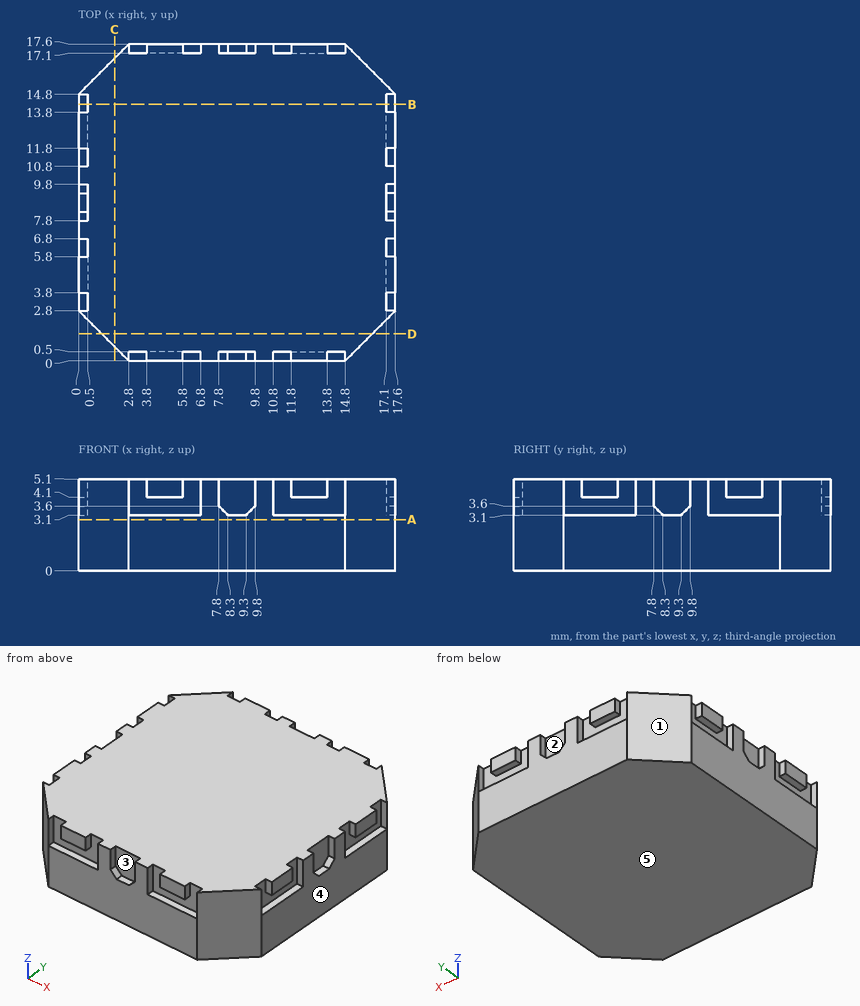
Geometry check sheet. Reference: drawing and pictorial views, mm from the part's lowest x, y, z. A direction names the side the tool comes from. Give positions to 0.01 mm unless a question says otherwise; leave off trailing zeros. Loops run counter-clockwise (first coordinate to the right, second up) from the corner with the lowest first, then second, coordinate; pieces in that order, holes last. Notation, with made-up numbers: (51.25, -10) - (59.25, -10) arc R11 cw to (59.25, 5) - close; hole circle Ø5 at (-20.5, 23). An arc over 180 degrees is marked (long way). One line per question, with ' | ' between items. Start each with the question number.
1. Cross-section at A-A, the plane z = 2.85. Enter the section's corners in (x, y), plus the area to 3 significant figures.
2. Gauge pin test, flat ends, axial feed: pin 1 Ø0.6 at (x, z) = (17.5, 4.5) entering from -Y; pin 2 Ø0.6 at (x, z) = (0.5, 4.5) entering from -Y. Record the tip position at first contact, or that the pin passes through.
3. Material ranges on line 1 along Y through (x, z) = (13.25, 3.6); line 2 along X through (y, z) = (2.25, 3.95); line 3 along X through (y, z) = (2, 1.8), recorded low to high. Write a range as [from, to].
4. Cross-section at C-C, the plane x = 2. Enter the section's corners in (y, z), plus the area to 3 significant figures.
5. Set-up check for the marked faces 1 and 2: record each of +Z, -Z, +X, -X, +Y, -Y from which the full face is reachable in a straight line by a thin tool's end or side.
6. Cross-section at D-D, the plane y = 1.5. Enter the section's corners in (x, z), plus the area to 3 significant figures.
7. Draft check along X on the marked faces 3, 4 and 5. Enter one of: released by +X, released by -X, zero draft, split by the parting line, or undercut.
8. Cross-section at B-B, the plane y = 14.25. Enter the section's corners in (x, z), plus the area to 3 significant figures.
Check result:
1) outline: (0, 2.8) - (2.8, 0) - (14.8, 0) - (17.6, 2.8) - (17.6, 14.8) - (14.8, 17.6) - (2.8, 17.6) - (0, 14.8) - close | area: 294 mm2
2) pin 1: stops at y = 2.4 | pin 2: stops at y = 2
3) line 1: y = [0.5, 17.1] | line 2: x = [0.55, 17.05] | line 3: x = [0.8, 16.8]
4) outline: (0.8, 0) - (16.8, 0) - (16.8, 5.1) - (0.8, 5.1) - close | area: 81.6 mm2
5) face 1: +Z, -Z, -X, +Y | face 2: +Z, +Y
6) outline: (1.3, 0) - (16.3, 0) - (16.3, 5.1) - (1.3, 5.1) - close | area: 76.5 mm2
7) face 3: undercut | face 4: released by +X | face 5: zero draft
8) outline: (0, 0) - (17.6, 0) - (17.6, 3.1) - (17.1, 3.1) - (17.1, 5.1) - (0.5, 5.1) - (0.5, 3.1) - (0, 3.1) - close | area: 87.8 mm2
